```python
from build123d import *

# Parameters (mm, degrees)
SKETCH1_W           = 25
SKETCH1_H           = 15
BOSS_EXTRUDE1_DEPTH = 20
SKETCH2_W           = 25
SKETCH2_H           = 14.55
CUT_EXTRUDE1_DEPTH  = 13
SKETCH4_R           = 2.55
BOSS_EXTRUDE2_DEPTH = 2
CHAMFER1_SIZE       = 1


with BuildPart() as part:
    # Sketch1 → Boss-Extrude1 (new body)
    with BuildSketch(Plane.XY):
        with Locations((12.5, 7.5)):
            Rectangle(SKETCH1_W, SKETCH1_H)
    extrude(amount=BOSS_EXTRUDE1_DEPTH)

    # Sketch2 → Cut-Extrude1 (cut)
    with BuildSketch(Plane.XZ):
        with Locations((12.5, 10)):
            Rectangle(SKETCH2_W, SKETCH2_H)
    extrude(amount=-CUT_EXTRUDE1_DEPTH, mode=Mode.SUBTRACT)

    # Sketch4 → Boss-Extrude2 (add)
    with BuildSketch(Plane(origin=(0, 15, 0), x_dir=(1, 0, 0), z_dir=(0, 1, 0))):
        with Locations(Location((12.5, -10, 0), (0, 0, 270))):
            Circle(SKETCH4_R)
    extrude(amount=BOSS_EXTRUDE2_DEPTH)

    # Chamfer1
    chamfer1_edges = [part.edges().sort_by_distance(p)[0] for p in [
        (12.5, 17, 7.45),
    ]]
    chamfer(chamfer1_edges, length=CHAMFER1_SIZE)


solid = part.part
```
CAD build for the part. Positions are in the model's coordinates, mm. A direction names the side the tool comes from. Round coordinates to 2 decimals unless told otherwise and drop trailing zeros. Loops run counter-clockwise (first coordinate to the right, second up) from the corner with the lowest first, then second, coordinate; pieces in that order, holes last. Notation, with made-up numbers: (26, -38) - (58, -38) arc R21 ccw to (58, -8) - close; hole circle Ø11 at (69.5, 71.5). An arc over 180 degrees is marked (long way). Return JSON: item names as keys, results as strings. Group by question number.
Q1. Band-saw the part on D-D on x = 12.5. Give the cut face in (y, z) (3 decimals).
Q2. Tool access for faces 1 (the face through (12, 6, 17.275)), 2 (the face through (25, 14, 9)): list every direction of +Z, -Z, +X, -X, +Y, -Y with a clear straight run to the whole face (end or side of a thin tool).
Q3. Flat gauge pins, fed straight in: pin 1 Ø7.5 at (x, z) = (16.5, 11.5) entering from -Y; pin 2 Ø6 at (y, z) = (2.5, 15) entering from -X. Where does each tip first touch, or does it go through?
Q4. Drill centre lines: line 1 along Z through (x, y) = (22, 7) (3 decimals); line 2 along Y through (x, z) = (9, 5.5); line 3 along Y through (x, z) = (13.25, 18). Where is each one in solid material? Low to high. Write a range as [from, to].
Q5. Band-saw the part on C-C on x = 22.75. Give the cut face in (y, z) (3 decimals).
Q6. Band-saw the part on B-B on z = 10. Give the cut face in (x, y), plus the area to 3 significant figures.
Q7. Two-plate mould, pull along Z, no slides. Class faces 3 (the face through (10.01, 15.49, 9.45)), 4 (the face through (12, 0, 19)), 5 (the face through (12, 6, 2.725)): +Z half, -Z half, draft (parallel to the pull), parting line (faces both ways), or undercut.
Q8. Band-saw the part on A-A on y = 3. Give the cut face in (x, z) (3 decimals), plus the area to 3 significant figures.
Solutions:
{
 "1": {"outline": "(0, 0) - (15, 0) - (15, 7.45) - (16, 7.45) - (17, 8.45) - (17, 11.55) - (16, 12.55) - (15, 12.55) - (15, 20) - (0, 20) - (0, 17.275) - (13, 17.275) - (13, 2.725) - (0, 2.725) - close"},
 "2": {"face 1": "+X, -X, -Y", "face 2": "+Z, -Z, +X, +Y, -Y"},
 "3": {"pin 1": "stops at y = 13", "pin 2": "stops at x = 0"},
 "4": {"line 1": "z = [0, 2.725], [17.275, 20]", "line 2": "y = [13, 15]", "line 3": "y = [0, 15]"},
 "5": {"outline": "(0, 0) - (15, 0) - (15, 20) - (0, 20) - (0, 17.275) - (13, 17.275) - (13, 2.725) - (0, 2.725) - close"},
 "6": {"outline": "(0, 13) - (25, 13) - (25, 15) - (15.05, 15) - (15.05, 16) - (14.05, 17) - (10.95, 17) - (9.95, 16) - (9.95, 15) - (0, 15) - close", "area": "59.2 mm^2"},
 "7": {"face 3": "parting line", "face 4": "draft", "face 5": "undercut"},
 "8": {"outline": "(0, 0) - (25, 0) - (25, 2.725) - (0, 2.725) - close; (0, 17.275) - (25, 17.275) - (25, 20) - (0, 20) - close", "area": "136 mm^2"}
}
